Check sheet for the modelled part. Datum: model origin and axes. Units: mm. A direction names the side the tool comes from. Coordinates: 2 decimals unless noted, no trailing zeros. Write each loop counter-clockwise with the first axis right and the second up, starting at its lowest first coordinate (ties: lowest second). Pieces come first, ordered by that corner, then holes. Notation, with made-up numbers: M 28.5,69 L 44.5,69 A28 cw 44.5,97 Z; hole C -14,33 d7. An arc over 180 degrees is marked long. Answer as CSV lines item,"result".
from build123d import *

# Parameters (mm, degrees)
EXTRUDE_1_DEPTH     = 1.2
CUT_EXTRUDE_START   = -1.2
CUT_EXTRUDE_1_DEPTH = 1.2
SKETCH_3_R          = 0.6
EXTRUDE_2_DEPTH     = 0.3
SKETCH_4_W          = 8.210741719
SKETCH_4_H          = 41.276753536
EXTRUDE_3_DEPTH     = 0.6


# Read off the part's stored shape, not the designer's step: Вырез-Вытянуть-Тонкостенный1
with BuildPart() as part:
    # Эскиз1 → Бобышка-Вытянуть1 (new body)
    with BuildSketch(Plane.XY):
        with BuildLine():
            Line((5.249737614, 19.025640721), (0.409977198, 22.613738961))
            Line((0.409977198, 22.613738961), (-7.294059401, 16.443030035))
            Line((-7.294059401, 16.443030035), (-5.378470688, -13.036872049))
            Line((-5.378470688, -13.036872049), (4.707402929, -22.613738961))
            Line((4.707402929, -22.613738961), (4.977734505, -22.318831787))
            add(Edge.make_bspline(
                [(4.977734505, -22.318831787), (5.380257217, -21.730973812), (6.179089351, -20.564331963), (6.904763741, -18.546948907), (7.294059401, -16.401738794), (7.239811, -14.930944587), (7.212045754, -14.178167322)],
                knots=[0, 0, 0, 0, 0.246766883, 0.489724704, 0.738832503, 1, 1, 1, 1], degree=3))
            Line((7.212045754, -14.178167322), (5.249737614, 19.025640721))
        make_face()
    extrude(amount=EXTRUDE_1_DEPTH)

    # Вырез-Вытянуть-Тонкостенный1 outline → Вырез-Вытянуть-Тонкостенный1 (cut)
    with BuildSketch(Plane.XY.offset(1.2).offset(CUT_EXTRUDE_START)):
        with BuildLine():
            Line((4.707402929, -22.613738961), (4.977734505, -22.318831787))
            add(Edge.make_bspline(
                [(4.977734505, -22.318831787), (5.380257217, -21.730973812), (6.179089351, -20.564331963), (6.904763741, -18.546948907), (7.294059401, -16.401738794), (7.239811, -14.930944587), (7.212045754, -14.178167322)],
                knots=[0, 0, 0, 0, 0.246766883, 0.489724704, 0.738832503, 1, 1, 1, 1], degree=3))
            Line((7.212045754, -14.178167322), (5.249737614, 19.025640721))
            Line((5.249737614, 19.025640721), (0.409977198, 22.613738961))
            Line((0.409977198, 22.613738961), (-7.294059401, 16.443030035))
            Line((-7.294059401, 16.443030035), (-5.378470688, -13.036872049))
            Line((-5.378470688, -13.036872049), (4.707402929, -22.613738961))
        make_face()
        with BuildLine():
            add(Edge.make_bspline(
                [(4.683954221, -22.039877798), (5.077205265, -21.465418253), (5.469505076, -20.890370995), (6.092414375, -19.640377114), (6.316902906, -18.988458608), (6.575666444, -17.98832874), (6.648049215, -17.650841196), (6.760734776, -16.966359137), (6.800621162, -16.619708847), (6.864229804, -15.582878491), (6.838032295, -14.890102205), (6.812480945, -14.197340575)],
                knots=[0, 0, 0, 0, 0.25, 0.25, 0.5, 0.5, 0.625, 0.625, 0.75, 0.75, 1, 1, 1, 1], degree=3))
            Line((4.683954221, -22.039877798), (-4.989468001, -12.854646977))
            Line((-4.989468001, -12.854646977), (-6.881392269, 16.261071759))
            Line((-6.881392269, 16.261071759), (0.419413416, 22.108804468))
            Line((0.419413416, 22.108804468), (4.861454817, 18.815566877))
            Line((4.861454817, 18.815566877), (6.812480945, -14.197340575))
        make_face(mode=Mode.SUBTRACT)
    extrude(amount=CUT_EXTRUDE_1_DEPTH, mode=Mode.SUBTRACT)

    # Эскиз3 → Бобышка-Вытянуть2 (add)
    with BuildSketch(Plane(origin=(5.952643232, 0.351794597, 0), x_dir=(0, 0, -1), z_dir=(0.9982582219819068, 0.05899595109430813, 0))):
        with Locations(Location((-0.6, 17.895988185, 0), (0, 0, 90))):
            Circle(SKETCH_3_R)
        with Locations((-0.6, 9.935988185)):
            Circle(SKETCH_3_R)
        with Locations((-0.6, 1.975988185)):
            Circle(SKETCH_3_R)
        with Locations((-0.6, -5.984011815)):
            Circle(SKETCH_3_R)
        with Locations((-0.6, -13.944011815)):
            Circle(SKETCH_3_R)
    extrude(amount=EXTRUDE_2_DEPTH)

    # Эскиз4 → Бобышка-Вытянуть3 (add)
    with BuildSketch(Plane(origin=(6.252120699, 0.369493382, 0), x_dir=(0, 0, -1), z_dir=(0.9982582219819068, 0.05899595109430812, 0))):
        with Locations((-0.847450423, 1.003287523)):
            Rectangle(SKETCH_4_W, SKETCH_4_H)
    extrude(amount=EXTRUDE_3_DEPTH)


solid = part.part
1) Section check A-A, the plane y = 0.5. Record the boundary of the cut face in (x, z), plus the area to 3 significant figures.
Answer key:
outline,"M -5.86,0 L 5.94,0 L 5.94,1.2 L -5.86,1.2 Z; M 6.24,-3.26 L 6.85,-3.26 L 6.85,4.95 L 6.24,4.95 Z"
area,"19.1 mm2"
2) Thickness scan on line 1 along Z through (x, y) = (1, -13); line 2 along X through (y, z) = (12, 0.75); line 3 along X through (y, z) = (10, 3.5). Record the ranges inside material, lowest first.
Answer key:
line 1,"z = 0 to 1.2"
line 2,"x = -6.6 to 5.26, 5.56 to 6.17"
line 3,"x = 5.68 to 6.28"
3) Section check B-B, the plane z = 2. Record the boundary of the cut face in (x, y), plus the area to 3 significant figures.
Answer key:
outline,"M 4.98,21.97 L 7.41,-19.23 L 8.01,-19.2 L 5.57,22.01 Z"
area,"24.8 mm2"
4) Section check C-C, the plane x = 1.25. Record the boundary of the cut face in (y, z), plus the area to 3 significant figures.
Answer key:
outline,"M -18.78,0 L 21.49,0 L 21.49,1.2 L -18.78,1.2 Z"
area,"48.3 mm2"
5) Depth check by flat-ended pin: P1, Ø4, axis at x = -4, y = 10, coming from the -Z side; P2, Ø2, axis at y = 11.5, z = 2.5, coming from the -X side; P3, Ø4, axis at x = -2.5, y = 9, coming from the +Z side. Enter the tip coordinate at first touch or a pass-through.
Answer key:
P1,"stops at z = 0"
P2,"stops at x = 5.54"
P3,"stops at z = 1.2"
6) Mould release check, pull along Y, two halves, no side actions. Record for faces 3 (the face through (5.13, 14.3, 0.59)), 4 (the face through (-5.922, 1.499, 0.592)), 5 (the face through (0, 0, 0)): pulls with the +Y half, pulls with the -Y half, needs draft (parallel to the pull), parting line crosses it, or undercut.
Answer key:
face 3,"undercut"
face 4,"pulls with the -Y half"
face 5,"needs draft"
7) Tool access check on faces 1 (the face through (6.775, 1.695, 0.905)), 2 (the face through (2.609, 20.485, 0.592)). Record the directions out of +Z, -Z, +X, -X, +Y, -Y that give a thin tool (end or side, any length) a straight path to the whole face; none if there is none.
Answer key:
face 1,"+Z, -Z, +X, +Y"
face 2,"+Z, -Z, +Y"
8) Section check D-D, the plane y = 15. Record the boundary of the cut face in (x, z).
Answer key:
outline,"M -6.8,0 L 5.09,0 L 5.09,1.2 L -6.8,1.2 Z; M 5.39,-3.26 L 5.99,-3.26 L 5.99,4.95 L 5.39,4.95 Z"
